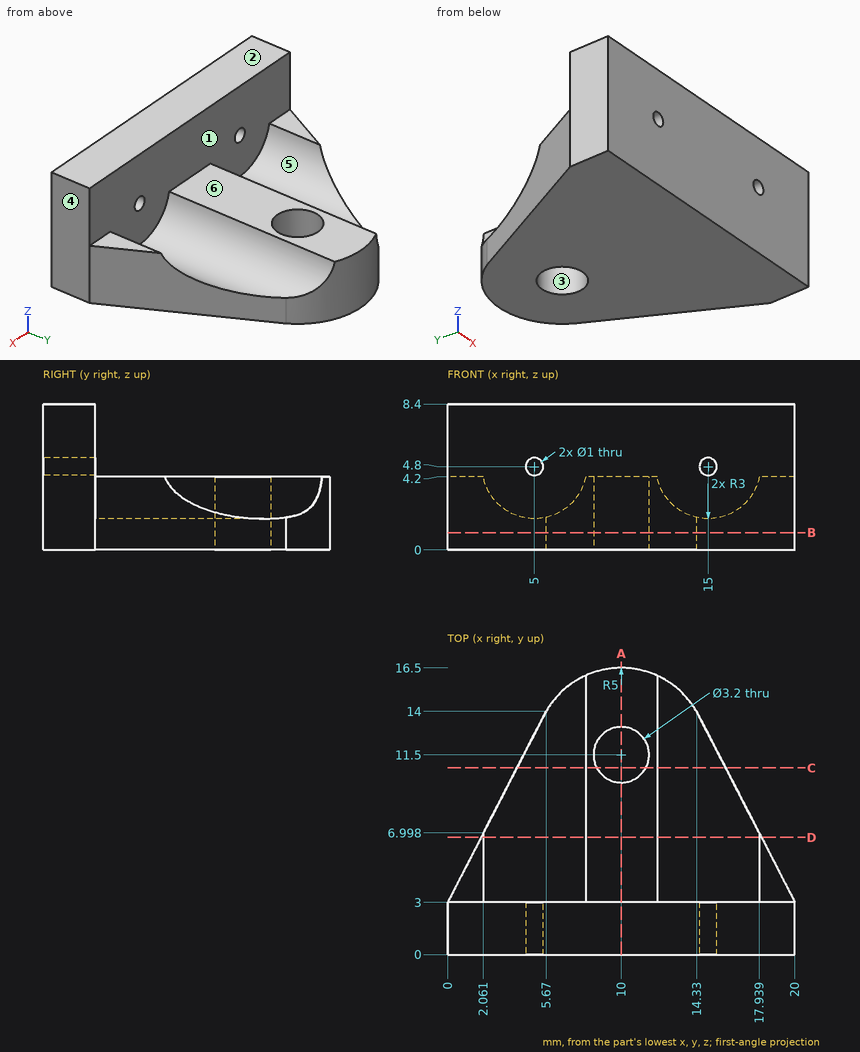
Geometry: see drawing. Coordinates: mm, zero at the bounding-box minimum. A direction names the side the tool comes from. Give positions to 0.01 mm unless a question says otherwise; leave off trailing zeros. Order: outer loops, then holes, each group sorted by start corner. A loop starts at its lowest first (then second) coordinate and runs counter-clockwise, first axis right, second up.
Q1. Set-up query: the marked faces 4, 5 and 6. Return all of +Z, -Z, +X, -X, +Y, -Y with unobstructed straight access to the full face (end or side cutting, diameter ignored); none if empty.
Checked values:
face 4: +Z, -Z, +X, +Y, -Y
face 5: +Z, +Y
face 6: +Z, +X, -X, +Y
Q2. Section B-B on z = 1. Output: boundary loops of the cut face in (x, y).
Checked values:
outline: (0, 0) - (20, 0) - (20, 3) - (14.33, 14) arc R5 ccw to (5.67, 14) - (0, 3) - close; hole circle Ø3.2 at (10, 11.5)
Q3. Section A-A on x = 10. Output: boundary loops of the cut face in (y, z).
Checked values:
outline: (0, 0) - (9.9, 0) - (9.9, 4.2) - (3, 4.2) - (3, 8.4) - (0, 8.4) - close; (13.1, 0) - (16.5, 0) - (16.5, 4.2) - (13.1, 4.2) - close
Q4. Section D-D on y = 6.75. Output: boundary loops of the cut face in (x, z).
Checked values:
outline: (1.93, 0) - (18.07, 0) - (18.07, 4.2) - (17.94, 4.2) arc R3 cw to (12.06, 4.2) - (7.94, 4.2) arc R3 cw to (2.06, 4.2) - (1.93, 4.2) - close
Q5. Section C-C on y = 10.75. Output: boundary loops of the cut face in (x, z) (1 decimal).
Checked values:
outline: (4, 0) - (8.6, 0) - (8.6, 4.2) - (7.9, 4.2) arc R3 cw to (4, 2) - close; (11.4, 0) - (16, 0) - (16, 2) arc R3 cw to (12.1, 4.2) - (11.4, 4.2) - close
Q6. Draft query along Y for the marked faces 1, 2 and 3. Return one class per face: +Y half, -Y half, draft (parallel to the pull), parting line (faces both ways), or undercut.
Checked values:
face 1: +Y half
face 2: draft
face 3: undercut
Q7. Contact query for flat-ended pins moving along their axis: pin 1 Ø1 at (x, z) = (9, 6) entering from +Y; pin 2 Ø2 at (y, z) = (14.5, 2.5) entering from +X; pin 3 Ø2 at (y, z) = (7, 1) entering from +X. Output: stop coordinate, or through.
Checked values:
pin 1: stops at y = 3
pin 2: stops at x = 14.46
pin 3: stops at x = 18.45
Q8. Ray query, probe 1 along Y at (x, z) = (10, 1.25); probe 2 along Y at (x, z) = (11, 7.75); probe 3 along Y at (x, z) = (13, 1.5). Return the intervals inside material, ascending.
Checked values:
probe 1: y = 0 to 9.9, 13.1 to 16.5
probe 2: y = 0 to 3
probe 3: y = 0 to 15.5
